from build123d import *

# Parameters (mm, degrees)
CASCA1_T                 = -0.9
RESSALTO_EXTRUS_O1_DEPTH = 9
FILETE1_R                = 1
ESBO_O3_R                = 2.38125
CORTE_EXTRUS_O1_DEPTH    = 39.143338529
SCALE1_SCALE             = 1.036484245


with BuildPart() as part:
    # Esboço1 → Revolução1 (revolve)
    with BuildSketch(Plane.XY, mode=Mode.PRIVATE) as revolu_o1_sk:
        Polygon((0, 0), (13.5, 0), (8.5, 4), (14, 10), (7.5, 15), (7.5, 24), (0, 24), align=None)
    revolve(revolu_o1_sk.sketch.rotate(Axis((0, 24, 0), (0, -1, 0)), 180), axis=Axis((0, 24, 0), (0, -1, 0)))

    # Casca1
    casca1_openings = [part.faces().sort_by_distance(p)[0] for p in [
        (0, 0, 0),
    ]]
    offset(amount=CASCA1_T, openings=casca1_openings, kind=Kind.INTERSECTION)

    # Esboço2 → Ressalto-extrusão1 (add)
    with BuildSketch(Plane(origin=(0, 24, 0), x_dir=(1, 0, 0), z_dir=(0, 1, 0))):
        Polygon((2.496763598, 3.885808136), (-2.11682676, 4.105164771), (-4.613590359, 0.219356636), (-2.496763598, -3.885808136), (2.11682676, -4.105164771), (4.613590359, -0.219356636), align=None)
    extrude(amount=RESSALTO_EXTRUS_O1_DEPTH)

    # Filete1
    filete1_edges = [part.edges().sort_by_distance(p)[0] for p in [
        (7.5, 15, 0),
        (14, 10, 0),
        (8.5, 4, 0),
    ]]
    fillet(filete1_edges, radius=FILETE1_R)

    # Esboço3 → Corte-extrusão1 (cut, through all)
    with BuildSketch(Plane(origin=(0, 33, 0), x_dir=(1, 0, 0), z_dir=(0, 1, 0))):
        with Locations(Location((0, 0, 0), (0, 0, 270))):
            Circle(ESBO_O3_R)
    extrude(amount=-CORTE_EXTRUS_O1_DEPTH, mode=Mode.SUBTRACT)


with BuildPart() as part_1:
    # Scale1: scaled about (0, 0, 0)
    add(part.part.scale(SCALE1_SCALE))


solid = part_1.part
Geometry: final body of the model. Coordinates: model frame, mm. A direction names the side the tool comes from. Give positions to 0.01 mm unless a question says otherwise; leave off trailing zeros. Write each loop counter-clockwise with the first axis right and the second up, starting at its lowest first coordinate (ties: lowest second). Pieces come first, ordered by that corner, then holes.
(1) Cut plane A-A, the plane y = 18.5. Return loops of the section in (x, z).
(2) Ray query, line 1 (Z direction, x = 0, y = 19); line 2 (Y direction, x = -9, z = 8.5); line 3 (Y direction, x = 9.25, z = 5.25). Return the intervals inside material, ascending.
(3) Access query for faces 1 (the conical face through (-9.072, 5.249, 3.762)), 2 (the flat face through (-3.47, 29.47, -2.27)), 3 (the flat face through (3.7, 29.47, -1.87)). Directions: +Z, -Z, +X, -X, +Y, -Y. A direction counts if a zero-diameter tool reaches every point of the face in a straight line with its end or side. Return the directions, or none.
(4) Cut plane D-D, the plane y = 7.5. Return loops of the section in (x, z), then the cut area to 3 significant figures.
(5) Mould query, pull axis Z, two halves, no side actions, for faces 4 (the flat face through (2, 34.204, 2)), 5 (the cylindrical face through (-3.157, 19.577, 6.069)), 6 (the conical face through (9.876, 3.286, -0.435)), 7 (the flat face through (-3, 23.943, 0)). Classes: released by +Z, released by -Z, zero draft, split by the parting line, or undercut.
(6) First-contact query: P1, Ø10, axis at x = -9.5, y = 22.5, coming from the +Z side; P2, Ø7, axis at x = 2.5, z = -2, coming from the -Y side; P3, Ø10, axis at x = 6, y = 6.5, coming from the +Z side. Flat tips, straight axial feed; report the tip coordinate or a pass-through.
(7) Cut plane B-B, the plane z = 10.25. Give the number of separate pieces and of enclosed holes in the cut face, then the cut area to 3 significant figures.
Values follow:
1. outline: circle Ø15.55 at (0, 0); hole circle Ø13.68 at (0, 0)
2. line 1: z = -7.77 to -6.84, 6.84 to 7.77
2. line 2: y = 0.1 to 1.29, 8.04 to 9.42, 10.83 to 12
2. line 3: y = 1.49 to 2.69, 6.14 to 7.52, 12.17 to 13.35
3. face 1: none
3. face 2: -Z, -X, +Y
3. face 3: -Z, +X, +Y
4. outline: circle Ø23.77 at (0, 0); hole circle Ø21.24 at (0, 0)
4. area: 89.5 mm2
5. face 4: zero draft
5. face 5: undercut
5. face 6: split by the parting line
5. face 7: undercut
6. P1: stops at z = 6.34
6. P2: stops at y = 23.94
6. P3: stops at z = 13.78
7. separate pieces: 2
7. enclosed holes: 1
7. area: 66.6 mm2
